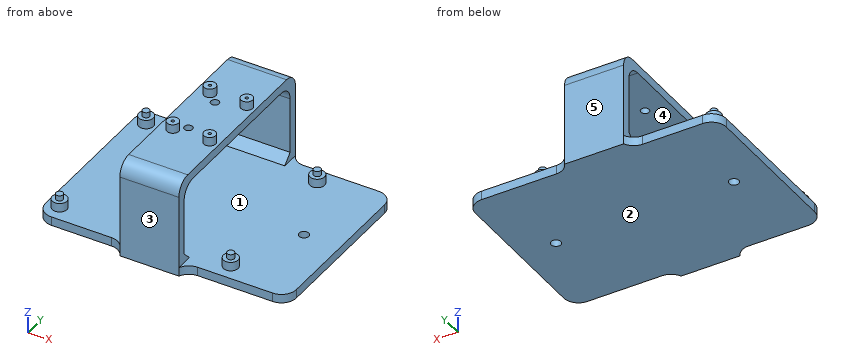
```python
from build123d import *

# Parameters (mm, degrees)
SKETCH1_W           = 85
SKETCH1_H           = 60
BOSS_EXTRUDE1_DEPTH = 3
SKETCH2_R           = 2.5
BOSS_EXTRUDE2_DEPTH = 3
SKETCH3_R           = 1.2
BOSS_EXTRUDE3_DEPTH = 1.8
SKETCH5_W           = 20
SKETCH5_H           = 30
BOSS_EXTRUDE4_DEPTH = 3
SKETCH6_W           = 20
SKETCH6_H           = 66
BOSS_EXTRUDE5_DEPTH = 3
SKETCH7_R           = 2
BOSS_EXTRUDE6_DEPTH = 3
SKETCH8_R           = 0.5
CUT_EXTRUDE2_DEPTH  = 5
SKETCH9_R           = 1.65
CUT_EXTRUDE3_DEPTH  = 3
FILLET1_R           = 5
CHAMFER1_SIZE       = 3
SKETCH10_R          = 1.4
CUT_EXTRUDE4_DEPTH  = 3


with BuildPart() as part:
    # Sketch1 → Boss-Extrude1 (new body)
    with BuildSketch(Plane.XY):
        Rectangle(SKETCH1_W, SKETCH1_H)
    extrude(amount=BOSS_EXTRUDE1_DEPTH)

    # Sketch2 → Boss-Extrude2 (add)
    with BuildSketch(Plane.XY.offset(3)):
        with Locations((-38, -24.5)):
            Circle(SKETCH2_R)
        with Locations((-38, 24.5)):
            Circle(SKETCH2_R)
        with Locations((20, 24.5)):
            Circle(SKETCH2_R)
        with Locations((20, -24.5)):
            Circle(SKETCH2_R)
    extrude(amount=BOSS_EXTRUDE2_DEPTH)

    # Sketch3 → Boss-Extrude3 (add)
    with BuildSketch(Plane.XY.offset(6)):
        with Locations((-38, 24.5)):
            Circle(SKETCH3_R)
        with Locations((20, 24.5)):
            Circle(SKETCH3_R)
        with Locations((-38, -24.5)):
            Circle(SKETCH3_R)
        with Locations((20, -24.5)):
            Circle(SKETCH3_R)
    extrude(amount=BOSS_EXTRUDE3_DEPTH)

    # Sketch5 → Boss-Extrude4 (add)
    with BuildSketch(Plane.XZ.offset(30)):
        with Locations((-2.5, 15)):
            Rectangle(SKETCH5_W, SKETCH5_H)
    boss_extrude4 = extrude(amount=BOSS_EXTRUDE4_DEPTH)

    # Mirror1: Boss-Extrude4 across plane
    add(boss_extrude4.mirror(Plane.ZX))

    # Sketch6 → Boss-Extrude5 (add)
    with BuildSketch(Plane.XY.offset(30)):
        with Locations((-2.5, 0)):
            Rectangle(SKETCH6_W, SKETCH6_H)
    extrude(amount=BOSS_EXTRUDE5_DEPTH)

    # Sketch7 → Boss-Extrude6 (add)
    with BuildSketch(Plane.XY.offset(33)):
        with Locations((-8, -10.5)):
            Circle(SKETCH7_R)
        with Locations((4.5, -10.5)):
            Circle(SKETCH7_R)
        with Locations((-8, 10.5)):
            Circle(SKETCH7_R)
        with Locations((4.5, 10.5)):
            Circle(SKETCH7_R)
    extrude(amount=BOSS_EXTRUDE6_DEPTH)

    # Sketch8 → Cut-Extrude2 (cut)
    with BuildSketch(Plane.XY.offset(36)):
        with Locations((-8, 10.5)):
            Circle(SKETCH8_R)
        with Locations((4.5, 10.5)):
            Circle(SKETCH8_R)
        with Locations((-8, -10.5)):
            Circle(SKETCH8_R)
        with Locations((4.5, -10.5)):
            Circle(SKETCH8_R)
    extrude(amount=-CUT_EXTRUDE2_DEPTH, mode=Mode.SUBTRACT)

    # Sketch9 → Cut-Extrude3 (cut)
    with BuildSketch(Plane.XY.offset(3)):
        with Locations((-30.15, 0)):
            Circle(SKETCH9_R)
        with Locations((30.15, 0)):
            Circle(SKETCH9_R)
    extrude(amount=-CUT_EXTRUDE3_DEPTH, mode=Mode.SUBTRACT)

    # Fillet1
    # the kernel refuses this fillet: 5 mm, written as the material it adds along each edge
    with BuildSketch(Plane(origin=(7.5, -30, 0), x_dir=(0, -1, 0), z_dir=(0, 0, 1)), Plane(origin=(-12.5, -30, 3), x_dir=(0, -1, 0), z_dir=(0, 0, -1))) as fillet1_piece_1:
        with BuildLine():
            CenterArc((5, 4.582575695), FILLET1_R, 180, 66.421821522)
            Line((0, 4.582575695), (0, 0))
            Line((0, 0), (3, 0))
        make_face()
    extrude(amount=3)
    with BuildSketch(Plane(origin=(-12.5, 30, 3), x_dir=(-1, 0, 0), z_dir=(0, 0, -1))) as fillet1_piece_2:
        with BuildLine():
            CenterArc((4.582575695, 5), FILLET1_R, 203.578178478, 66.421821522)
            Line((0, 3), (0, 0))
            Line((0, 0), (4.582575695, 0))
        make_face()
    extrude(amount=3)
    with BuildSketch(Plane(origin=(7.5, 30, 0), x_dir=(0, 1, 0), z_dir=(0, 0, 1))) as fillet1_piece_3:
        with BuildLine():
            CenterArc((5, -4.582575695), FILLET1_R, 113.578178478, 66.421821522)
            Line((0, -4.582575695), (0, 0))
            Line((0, 0), (3, 0))
        make_face()
    extrude(amount=3)
    with BuildSketch(Plane(origin=(7.5, -30, 30), x_dir=(0, 1, 0), z_dir=(-1, 0, 0)), Plane(origin=(7.5, 30, 30), x_dir=(0, 0, -1), z_dir=(-1, 0, 0))) as fillet1_piece_4:
        with BuildLine():
            CenterArc((FILLET1_R, FILLET1_R), FILLET1_R, 180, 90)
            Line((0, FILLET1_R), (0, 0))
            Line((0, 0), (FILLET1_R, 0))
        make_face()
    extrude(amount=20)
    # the kernel refuses this fillet: 5 mm, written as the material it takes off along each edge
    with BuildSketch(Plane(origin=(42.5, 30, -12.5), x_dir=(-1, 0, 0), z_dir=(0, 0, 1)), Plane(origin=(42.5, -30, -12.5), x_dir=(0, 1, 0), z_dir=(0, 0, 1))) as fillet1_2_piece_1:
        with BuildLine():
            CenterArc((FILLET1_R, FILLET1_R), FILLET1_R, 180, 90)
            Line((0, FILLET1_R), (0, 0))
            Line((0, 0), (FILLET1_R, 0))
        make_face()
    extrude(amount=28, mode=Mode.SUBTRACT)
    with BuildSketch(Plane(origin=(-42.5, 30, -12.5), x_dir=(1, 0, 0), z_dir=(0, 0, 1)), Plane(origin=(-42.5, -30, -12.5), x_dir=(0, 1, 0), z_dir=(0, 0, 1))) as fillet1_2_piece_2:
        with BuildLine():
            CenterArc((FILLET1_R, -FILLET1_R), FILLET1_R, 90, 90)
            Line((0, -FILLET1_R), (0, 0))
            Line((0, 0), (FILLET1_R, 0))
        make_face()
    extrude(amount=28, mode=Mode.SUBTRACT)
    with BuildSketch(Plane(origin=(20, -33, 33), x_dir=(0, 0, -1), z_dir=(-1, 0, 0)), Plane(origin=(-25, 33, 33), x_dir=(0, 0, -1), z_dir=(1, 0, 0))) as fillet1_2_piece_3:
        with BuildLine():
            CenterArc((FILLET1_R, -FILLET1_R), FILLET1_R, 90, 90)
            Line((0, -FILLET1_R), (0, 0))
            Line((0, 0), (FILLET1_R, 0))
        make_face()
    extrude(amount=45, mode=Mode.SUBTRACT)

    # Chamfer1
    chamfer1_edges = [part.edges().sort_by_distance(p)[0] for p in [
        (-2.5, -30, 3),
        (-2.5, 30, 3),
    ]]
    chamfer(chamfer1_edges, length=CHAMFER1_SIZE)

    # Sketch10 → Cut-Extrude4 (cut)
    with BuildSketch(Plane(origin=(0, 0, 30), x_dir=(-1, 0, 0), z_dir=(0, 0, -1))):
        with Locations((4.5, -7.5)):
            Circle(SKETCH10_R)
        with Locations((4.5, 7.5)):
            Circle(SKETCH10_R)
    extrude(amount=-CUT_EXTRUDE4_DEPTH, mode=Mode.SUBTRACT)


solid = part.part
```
Part model, mm, in its own coordinate system. Face numbers are marked on the shaded views. A direction names the side the tool comes from. Coordinates: 2 decimals unless noted, no trailing zeros. Write each loop counter-clockwise with the first axis right and the second up, starting at its lowest first coordinate (ties: lowest second). Pieces come first, ordered by that corner, then holes.
Item 1: Probe line 1 (Y direction, x = 4.5, z = 33.25); line 2 (Z direction, x = 5, y = -23.5); line 3 (Y direction, x = -4, z = 31). List the from-to ranges inside material, lowest first.
Item 2: Slice it at D-D (y = -7.5). Write the cut outline in (x, z).
Item 3: Which spindle directions (+Z, -Z, +X, -X, +Y, -Y) get a long thin tool onto all of the face, cutting with end or side? Do the marked faces 4 and 5. Say none if no direction does.
Item 4: Slice it at C-C (z = 9). Write the cut outline in (x, y), and give its area (3 significant figures).
Item 5: Slice it at B-B (y = 0). Write the cut outline in (x, z).
Item 6: Pin check, flat tips, straight feed: pin 1 (1.5 mm diameter, centred on x = 24.5, z = 2, fed in from -Y); pin 2 (3 mm diameter, centred on x = 12.5, y = -19, fed in from -Z); pin 3 (10 mm diameter, centred on y = 16.5, z = 9.5, fed in from -X); pin 4 (5.5 mm diameter, centred on x = 21, y = -24, fed in from +Z). Stop position of each tip, or through.
Item 7: Slice it at A-A (x = -30.15). Write the cut outline in (y, z), and give its area (3 significant figures).
Item 8: Mould opens along Z. For the marked faces 1, 2 and 3 say: released by +Z, released by -Z, zero draft, split by the parting line, or undercut.
Results found:
1. line 1: y = -12.5 to -11, -10 to -8.5, 8.5 to 10, 11 to 12.5
1. line 2: z = 0 to 3, 30 to 33
1. line 3: y = -32 to -8.81, -6.19 to 6.19, 8.81 to 32
2. outline: (-42.5, 0) - (42.5, 0) - (42.5, 3) - (-42.5, 3) - close; (-12.5, 30) - (-5.9, 30) - (-5.9, 33) - (-12.5, 33) - close; (-3.1, 30) - (7.5, 30) - (7.5, 33) - (-3.1, 33) - close
3. face 4: +X, -X
3. face 5: +Z, -Z, +X, -X, +Y
4. outline: (-12.5, -33) - (7.5, -33) - (7.5, -30) - (-12.5, -30) - close; (-12.5, 30) - (7.5, 30) - (7.5, 33) - (-12.5, 33) - close
4. area: 120 mm2
5. outline: (-42.5, 0) - (-31.8, 0) - (-31.8, 3) - (-42.5, 3) - close; (-28.5, 0) - (28.5, 0) - (28.5, 3) - (-28.5, 3) - close; (-12.5, 30) - (7.5, 30) - (7.5, 33) - (-12.5, 33) - close; (31.8, 0) - (42.5, 0) - (42.5, 3) - (31.8, 3) - close
6. pin 1: stops at y = -30
6. pin 2: stops at z = 0
6. pin 3: passes through
6. pin 4: stops at z = 7.8
7. outline: (-30, 0) - (-1.65, 0) - (-1.65, 3) - (-30, 3) - close; (1.65, 0) - (30, 0) - (30, 3) - (1.65, 3) - close
7. area: 170 mm2
8. face 1: undercut
8. face 2: released by -Z
8. face 3: zero draft
